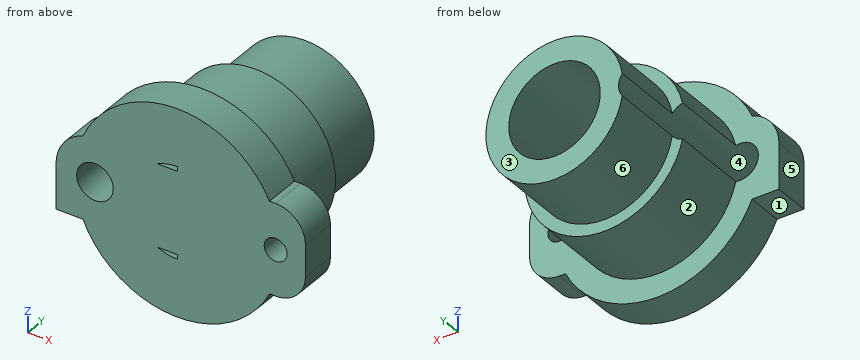
```python
from build123d import *

# Parameters (mm, degrees)
SKETCH_9_W          = 53
SKETCH_9_H          = 36
EXTRUDE_1_DEPTH     = 16
SKETCH_10_W         = 56
SKETCH_10_H         = 40
EXTRUDE_2_DEPTH     = 16
SKETCH_11_R         = 8
CUT_EXTRUDE_3_DEPTH = 82
SKETCH_12_R         = 5
CUT_EXTRUDE_6_DEPTH = 82
FILLET_1_R          = 17
FILLET_2_R          = 13


with BuildPart() as part:
    # 草图8 → 旋转1 (revolve)
    with BuildSketch(Plane.XY, mode=Mode.PRIVATE) as revolve_1_sk:
        Polygon((20, 0), (45, 0), (45, 16), (35, 16), (35, 50), (30, 50), (30, 82), (20, 82), align=None)
    revolve(revolve_1_sk.sketch.rotate(Axis((0, -10, 0), (0, 1, 0)), 90), axis=Axis((0, -10, 0), (0, 1, 0)))

    # 草图9 → 凸台-拉伸1 (add)
    with BuildSketch(Plane(origin=(0, 0, 0), x_dir=(1, 0, 0), z_dir=(0, 1, 0))):
        with Locations((-26.5, 0)):
            Rectangle(SKETCH_9_W, SKETCH_9_H)
    extrude(amount=EXTRUDE_1_DEPTH)

    # 草图10 → 凸台-拉伸2 (add)
    with BuildSketch(Plane(origin=(0, 0, 0), x_dir=(1, 0, 0), z_dir=(0, 1, 0))):
        with Locations((28, 0)):
            Rectangle(SKETCH_10_W, SKETCH_10_H)
    extrude(amount=EXTRUDE_2_DEPTH)

    # 草图11 → 切除-拉伸3 (cut)
    with BuildSketch(Plane(origin=(0, 0, 0), x_dir=(1, 0, 0), z_dir=(0, 1, 0))):
        with Locations(Location((-36, 0, 0), (0, 0, 76.445215963))):
            Circle(SKETCH_11_R)
    extrude(amount=CUT_EXTRUDE_3_DEPTH, mode=Mode.SUBTRACT)

    # 草图12 → 切除-拉伸6 (cut)
    with BuildSketch(Plane(origin=(0, 0, 0), x_dir=(1, 0, 0), z_dir=(0, 1, 0))):
        with Locations(Location((43, 0, 0), (0, 0, 270))):
            Circle(SKETCH_12_R)
    extrude(amount=CUT_EXTRUDE_6_DEPTH, mode=Mode.SUBTRACT)

    # 圆角1
    # the kernel refuses this fillet: 17 mm, written as the material it takes off along each edge
    with BuildSketch(Plane(origin=(-53, -40.428103648, 18), x_dir=(0, 0, -1), z_dir=(0, 1, 0))) as fillet_1_piece_1:
        with BuildLine():
            CenterArc((16.171241459, -17), FILLET_1_R, 90, 72.035815704)
            Line((0, -11.756818745), (-0.323424829, -11.65195512))
            ThreePointArc((-0.323424829, -11.65195512), (-0.34, -5.878409373), (-0.34, 0))
            Line((-0.34, 0), (0, 0.34))
            Line((0, 0.34), (16.171241459, 0.34))
            Line((16.171241459, 0.34), (16.171241459, 0))
        make_face()
    extrude(amount=96.856207296, mode=Mode.SUBTRACT)

    # 圆角2
    fillet_2_edges = [part.edges().sort_by_distance(p)[0] for p in [
        (56, 8, 20),
        (56, 8, -20),
    ]]
    fillet(fillet_2_edges, radius=FILLET_2_R)


solid = part.part
```
Geometry check sheet. Reference: the model listing, model coordinates, mm. Face numbers are marked on the shaded views. A direction names the side the tool comes from. Coordinates: 2 decimals unless noted, no trailing zeros. Loops run counter-clockwise (first coordinate to the right, second up) from the corner with the lowest first, then second, coordinate; pieces in that order, holes last. Notation, with made-up numbers: (-35.5, 39) -> (-28.5, 39) arc R27 cw to (-28.5, 65) -> close; hole circle Ø8 at (20.5, 78.5). An arc over 180 degrees is marked (long way). Put each result on its own line as item: value.
1) Gauge pin test, flat ends, axial feed: pin 1 Ø0.6 at (y, z) = (11.5, -18.5) entering from -X; pin 2 Ø4 at (x, y) = (5.5, 52.5) entering from -Z; pin 3 Ø12 at (y, z) = (34.5, -30) entering from -X; pin 4 Ø9.5 at (x, z) = (-36, 0) entering from +Y. Record the tip position at first contact, or that the pin passes through.
Result set:
pin 1: stops at x = -41.16
pin 2: stops at z = -29.8
pin 3: stops at x = -25.48
pin 4: passes through
2) Cross-section at B-B on x = 32. Record the boundary of the cut face in (y, z).
Result set:
outline: (0, -31.64) -> (16, -31.64) -> (16, -14.18) -> (50, -14.18) -> (50, 14.18) -> (16, 14.18) -> (16, 31.64) -> (0, 31.64) -> close
3) Cross-section at A-A on z = 0. Record the boundary of the cut face in (x, y).
Result set:
outline: (-53, 0) -> (-44, 0) -> (-44, 16) -> (-53, 16) -> close; (-28, 0) -> (38, 0) -> (38, 16) -> (35, 16) -> (35, 50) -> (30, 50) -> (30, 82) -> (20, 82) -> (20, 16) -> (-20, 16) -> (-20, 82) -> (-28, 82) -> close; (48, 0) -> (56, 0) -> (56, 16) -> (48, 16) -> close
4) Cross-section at D-D on x = -18. Record the boundary of the cut face in (y, z).
Result set:
outline: (0, -41.24) -> (16, -41.24) -> (16, -30.02) -> (50, -30.02) -> (50, -24) -> (82, -24) -> (82, -8.72) -> (16, -8.72) -> (16, 8.72) -> (82, 8.72) -> (82, 24) -> (50, 24) -> (50, 30.02) -> (16, 30.02) -> (16, 41.24) -> (0, 41.24) -> close
5) Thickness scan on line 1 (X direction, y = 4.5, z = 0); line 2 (Z direction, x = 0, y = 62); line 3 (Z direction, x = 43, y = 12.75). Record the ranges inside material, lowest first.
Result set:
line 1: x = -53 to -44, -28 to 38, 48 to 56
line 2: z = -30 to -20, 20 to 30
line 3: z = -20 to -5, 5 to 20
6) Tool access check on the marked faces 5 and 6. Record the directions out of +Z, -Z, +X, -X, +Y, -Y that give a thin tool (end or side, any length) a straight path to the whole face; none if there is none.
Result set:
face 5: +Z, -Z, -X, +Y, -Y
face 6: +Y
7) Release check for a two-part mould opening along Z. For the marked faces 1, 2, 3 and 4 record: released by +Z, released by -Z, zero draft, split by the parting line, or undercut.
Result set:
face 1: released by -Z
face 2: split by the parting line
face 3: zero draft
face 4: undercut
8) Cross-section at C-C on y = 61. Record the boundary of the cut face in (x, z), plus the area to 3 significant figures.
Result set:
outline: (-29.61, -4.81) arc R30 ccw (long way) to (-29.61, 4.81) arc R8 cw to start; hole circle Ø40 at (0, 0)
area: 1,560 mm^2
